```python
from build123d import *

# Parameters (mm, degrees)
F0_W         = 68
F0_H         = 24.8
F0_W_2       = 62
F0_H_2       = 18
F1_DEPTH     = 35
F0_H_3       = 5
F2_DEPTH     = 12
F3_R         = 6.7597979746
F4_R         = 6.7597979746
F5_R         = 4.99999
F6_R         = 4.99999
F7_T1_DEPTH  = 62
F8_T1_DEPTH  = 62
F9_T4_DEPTH  = 47.7128784748
F9_S5_R      = 5.0000000001
F9_T6_DEPTH  = 26
F9_S7_R      = 5.0000000001
F9_T8_DEPTH  = 26
F10_T4_DEPTH = 47.7128784748
F10_S5_R     = 5.0000000001
F10_T6_DEPTH = 26
F10_S7_R     = 5.0000000001
F10_T8_DEPTH = 26


# Not quite as in the source:
# - a fillet or chamfer that OpenCascade refuses, or shapes differently, is made with other operations: its cross-section is extruded or revolved along the edge and cut away or added
# - a fillet or chamfer is up to 0.001 mm smaller than in the source, because OpenCascade refuses the exact size


with BuildPart() as f1:
    # F0 (on Top) → F1 (new body)
    with BuildSketch(Plane.XY):
        Rectangle(F0_W, F0_H)
        Rectangle(F0_W_2, F0_H_2, mode=Mode.SUBTRACT)
    extrude(amount=F1_DEPTH)

    # F0 (on Top) → F2 (join)
    with BuildSketch(Plane.XY):
        with Locations((0, 14.9)):
            Rectangle(F0_W, F0_H_3)
        with Locations((0, -14.9)):
            Rectangle(F0_W, F0_H_3)
    extrude(amount=F2_DEPTH)

    # F3
    f3_edges = [f1.edges().sort_by_distance(p)[0] for p in [
        (0, 9, 0),
    ]]
    fillet(f3_edges, radius=F3_R)

    # F4
    f4_edges = [f1.edges().sort_by_distance(p)[0] for p in [
        (0, -9, 0),
    ]]
    fillet(f4_edges, radius=F4_R)

    # F5 (radius 5 in the source; OpenCascade refuses exactly that, so slightly less here)
    f5_edges = [f1.edges().sort_by_distance(p)[0] for p in [
        (0, 17.4, 12),
    ]]
    fillet(f5_edges, radius=F5_R)

    # F6 (radius 5 in the source; OpenCascade refuses exactly that, so slightly less here)
    f6_edges = [f1.edges().sort_by_distance(p)[0] for p in [
        (0, -17.4, 12),
    ]]
    fillet(f6_edges, radius=F6_R)

    # F7: fillet of radius 5 on 1 edges, made by hand

    # F7_s2 → F7_t1 (cut)
    with BuildSketch(Plane.YZ.offset(-31)):
        with BuildLine():
            ThreePointArc((14, 35), (10.4644660941, 33.5355339059), (9, 30))
            Line((9, 30), (9, 35))
            Line((9, 35), (14, 35))
        make_face()
    extrude(amount=F7_T1_DEPTH, mode=Mode.SUBTRACT)

    # F8: fillet of radius 5 on 1 edges, made by hand

    # F8_s2 → F8_t1 (cut)
    with BuildSketch(Plane.YZ.offset(-31)):
        with BuildLine():
            ThreePointArc((-9, 30), (-10.4644660941, 33.5355339059), (-14, 35))
            Line((-14, 35), (-9, 35))
            Line((-9, 35), (-9, 30))
        make_face()
    extrude(amount=F8_T1_DEPTH, mode=Mode.SUBTRACT)

    # F9: fillet of radius 5 on 1 edges, made by hand


with BuildPart() as f9_tool2:
    # F9_s3 → F9_t4 (new body)
    with BuildSketch(Plane.XZ.offset(-23.8564392374)):
        with BuildLine():
            ThreePointArc((-31, 30.417424305), (-31.8166998673, 33.1560370926), (-34, 35))
            Line((-34, 35), (-31, 35))
            Line((-31, 35), (-31, 30.417424305))
        make_face()
    extrude(amount=F9_T4_DEPTH)

    # F9_s5 → F9_t6 (cut, symmetric)
    with BuildSketch(Plane.YZ.offset(-32.5)):
        with Locations((-14.0000000001, 29.9999999999)):
            Circle(F9_S5_R)
    extrude(amount=F9_T6_DEPTH, both=True, mode=Mode.SUBTRACT)

    # F9_s7 → F9_t8 (cut, symmetric)
    with BuildSketch(Plane.YZ.offset(-32.5)):
        with Locations((14.0000000001, 29.9999999999)):
            Circle(F9_S7_R)
    extrude(amount=F9_T8_DEPTH, both=True, mode=Mode.SUBTRACT)


with BuildPart() as f1_1:
    add(f1.part)

    # F9_t1: cut F9_tool2
    add(f9_tool2.part, mode=Mode.SUBTRACT)

    # F10: fillet of radius 5 on 1 edges, made by hand


with BuildPart() as f10_tool2:
    # F10_s3 → F10_t4 (new body)
    with BuildSketch(Plane.XZ.offset(-23.8564392374)):
        with BuildLine():
            ThreePointArc((31, 30.417424305), (31.8166998673, 33.1560370926), (34, 35))
            Line((34, 35), (31, 35))
            Line((31, 35), (31, 30.417424305))
        make_face()
    extrude(amount=F10_T4_DEPTH)

    # F10_s5 → F10_t6 (cut, symmetric)
    with BuildSketch(Plane.YZ.offset(32.5)):
        with Locations((-14.0000000001, 29.9999999999)):
            Circle(F10_S5_R)
    extrude(amount=F10_T6_DEPTH, both=True, mode=Mode.SUBTRACT)

    # F10_s7 → F10_t8 (cut, symmetric)
    with BuildSketch(Plane.YZ.offset(32.5)):
        with Locations((14.0000000001, 29.9999999999)):
            Circle(F10_S7_R)
    extrude(amount=F10_T8_DEPTH, both=True, mode=Mode.SUBTRACT)


with BuildPart() as f1_2:
    add(f1_1.part)

    # F10_t1: cut F10_tool2
    add(f10_tool2.part, mode=Mode.SUBTRACT)


solid = f1_2.part
```
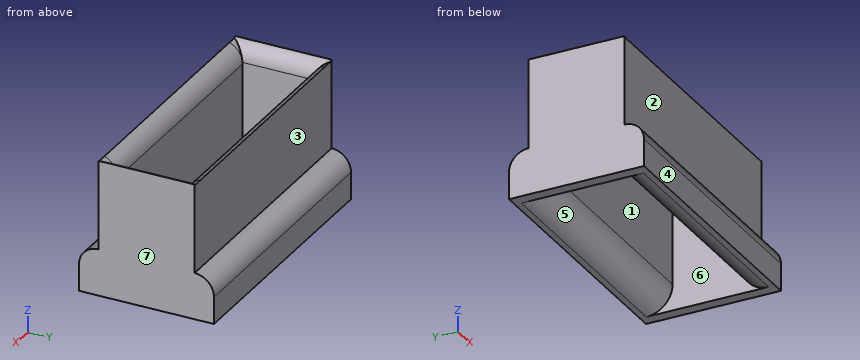
Geometry check sheet. Reference: the model listing, model coordinates, mm. Face numbers are marked on the shaded views. A direction names the side the tool comes from. Round coordinates to 2 decimals unless told otherwise and drop trailing zeros. Loops run counter-clockwise (first coordinate to the right, second up) from the corner with the lowest first, then second, coordinate; pieces in that order, holes last. Notation, with made-up numbers: M 73.5,-30.75 L 92.5,-30.75 A9 ccw 92.5,-17.75 Z; hole C 51.25,52.25 d4. An arc over 180 degrees is marked long. Return JSON: item names as keys, results as strings. Group by question number.
(1) Mould release check, pull along Y, two halves, no side actions. Record for the marked faces 4, 5, 6 and 7: pulls with the +Y half, pulls with the -Y half, needs draft (parallel to the pull), parting line crosses it, or undercut.
(2) Section check C-C, the plane y = 15. Enter the section's corners in (x, z).
(3) Set-up check for the marked faces 1, 2 and 3: record each of +Z, -Z, +X, -X, +Y, -Y from which the full face is reachable in a straight line by a thin tool's end or side.
(4) Section check A-A, the plane z = 18. Enter the section's corners in (x, y), and give its area (3 significant figures).
(5) Go/stop test with flat-tipped pins: pin 1 (10 mm diameter, centred on x = -14, z = 23, fed in from +Y); pin 2 (11.5 mm diameter, centred on x = -12, z = 13.5, fed in from -Y); pin 3 (2 mm diameter, centred on x = -9.5, z = 27.5, fed in from -Y). Record where each tip stops, or that it passes through.
(6) Section check D-D, the plane z = 9.5. Enter the section's corners in (x, y), and give its area (3 significant figures).
(7) Scan lines: line 1 along X through (y, z) = (-8, 4); line 2 along Y through (x, z) = (-18, 20); line 3 along Y through (x, z) = (11.5, 7). Record each from-to range of solid material in increasing order. Write a range as [from, to].
Data:
{
 "1": {"face 4": "pulls with the -Y half", "face 5": "undercut", "face 6": "undercut", "face 7": "needs draft"},
 "2": {"outline": "M -34,0 L -31,0 L -31,0.04 L 31,0.04 L 31,0 L 34,0 L 34,11.27 L -34,11.27 Z"},
 "3": {"face 1": "+Z, -Z", "face 2": "+Z, +X, -X, -Y", "face 3": "+Z, +X, -X, +Y"},
 "4": {"outline": "M -34,-12.4 L 34,-12.4 L 34,12.4 L -34,12.4 Z; hole M -31,-9 L 31,-9 L 31,9 L -31,9 Z", "area": "570 mm²"},
 "5": {"pin 1": "y = 12.4", "pin 2": "y = -17.34", "pin 3": "y = -12.4"},
 "6": {"outline": "M -34,-16.73 L 34,-16.73 L 34,16.73 L -34,16.73 Z; hole M -31,-9 L 31,-9 L 31,9 L -31,9 Z", "area": "1,160 mm²"},
 "7": {"line 1": "[-34, -31], [31, 34]", "line 2": "[-12.4, -9], [9, 12.4]", "line 3": "[-17.4, -9], [9, 17.4]"}
}
